Check sheet for the modelled part. Datum: model origin and axes. Units: mm. Round coordinates to 2 decimals unless told otherwise and drop trailing zeros. Write each loop counter-clockwise with the first axis right and the second up, starting at its lowest first coordinate (ties: lowest second). Pieces come first, ordered by that corner, then holes. Notation, with made-up numbers: (67.25, -15.5) -> (106.25, -15.5) arc R25 cw to (106.25, 10.5) -> close; hole circle Ø2 at (-2, -31.5). An arc over 180 degrees is marked (long way). Write item = value, one per line.
from build123d import *

# Parameters (mm, degrees)
EXTRUDE_1_DEPTH     = 3
SKETCH_2_R          = 1.15
CUT_EXTRUDE_1_DEPTH = 291.058614766


with BuildPart() as part:
    # 草图1 → 凸台-拉伸1 (new body)
    with BuildSketch(Plane.XY):
        Polygon((0, 0), (10, 5), (280, 5), (290, 0), (280, 0), (280, -3), (255, -3), (255, 0), (245, 0), (245, -3), (220, -3), (220, 0), (210, 0), (210, -3), (185, -3), (185, 0), (175, 0), (175, -3), (150, -3), (150, 0), (140, 0), (140, -3), (115, -3), (115, 0), (105, 0), (105, -3), (80, -3), (80, 0), (70, 0), (70, -3), (45, -3), (45, 0), (35, 0), (35, -3), (10, -3), (10, 0), align=None)
    extrude(amount=EXTRUDE_1_DEPTH)

    # 草图2 → 切除-拉伸1 (cut, through all)
    with BuildSketch(Plane.XY.offset(3)):
        with Locations((22.5, 2.85)):
            Circle(SKETCH_2_R)
        with Locations((57.5, 2.85)):
            Circle(SKETCH_2_R)
        with Locations((92.5, 2.85)):
            Circle(SKETCH_2_R)
        with Locations((127.5, 2.85)):
            Circle(SKETCH_2_R)
        with Locations((162.5, 2.85)):
            Circle(SKETCH_2_R)
        with Locations((197.5, 2.85)):
            Circle(SKETCH_2_R)
        with Locations((232.5, 2.85)):
            Circle(SKETCH_2_R)
        with Locations((267.5, 2.85)):
            Circle(SKETCH_2_R)
    extrude(amount=-CUT_EXTRUDE_1_DEPTH, mode=Mode.SUBTRACT)


solid = part.part
(1) Go/stop test with flat-tipped pins: P1, Ø3.5, axis at x = 232.5, y = 2.85, coming from the +Z side; P2, Ø0.9, axis at y = -2, z = 1.5, coming from the +X side; P3, Ø1, axis at y = 2, z = 2, coming from the +X side; P4, Ø1.5, axis at x = 285, z = 1, coming from the -Y side. Record where each tip stops, or that it passes through.
Worked answers:
P1 = 3
P2 = 280
P3 = 287
P4 = 0
(2) Sectioned sample at A-A on y = -1.75. Count the separate pieces of the cut face and the enclosed holes in it, then the cut area to 3 significant figures.
Worked answers:
separate_pieces = 8
enclosed_holes = 0
area = 600 mm²
(3) Sectioned sample at C-C on x = 217. Enter the section's corners in (y, z), then the cut area to 3 significant figures.
Worked answers:
outline = (0, 0) -> (5, 0) -> (5, 3) -> (0, 3) -> close
area = 15.0 mm²
(4) Material ranges on L1, parallel to Y at x = 92.5, z = 1.2; L2, parallel to Y at x = 73, z = 0.35; L3, parallel to X at y = 0.75, z = 1.7, recorded low to high. Write a range as [from, to].
Worked answers:
L1 = [-3, 1.7], [4, 5]
L2 = [0, 5]
L3 = [1.5, 288.5]
